For this review, take the finished solid that the model builds, in its own axes (mm). Face numbers are marked on the shaded views. A direction names the side the tool comes from. Give positions to 0.01 mm unless a question says otherwise; leave off trailing zeros. Write each loop counter-clockwise with the first axis right and the second up, starting at its lowest first coordinate (ties: lowest second). Pieces come first, ordered by that corner, then holes.
1) Draft analysis for pull direction Z (two halves, no side actions). For the marked faces 4, 5, 6 and 7, state which applies: pulls with the +Z half, pulls with the -Z half, needs draft (parallel to the pull), parting line crosses it, or undercut.
2) Wall thickness on line 1 along Y through (x, z) = (-24, 11); line 2 along X through (y, z) = (-27, 26.5); line 3 along X through (y, z) = (-14, 32): over which ranges is each line inside the solid? List them lowest first.
3) We need section C-C on x = -18.25. Give the boundary of the cut face in (y, z), and give its area (3 significant figures).
4) We need section B-B on z = 11. Give the boundary of the cut face in (x, y), and give its area (3 significant figures).
5) We need section D-D on y = -26.5. Give the boundary of the cut face in (x, z).
6) For P1, Ø3, axis at x = -16.5, y = -8.5, coming from the +Z side; P2, Ø12, axis at y = -13, z = 28, coming from the -X side; P3, Ø1, axis at y = -11, z = 10, coming from the -X side, all flat-tipped, find the tip position at first contact; note any pin that passes through.
7) Machinability: for the marked faces 1, 2 and 3, which of the approach directions +Z, -Z, +X, -X, +Y, -Y give a long, thin tool a straight path to every point of the face, cutting with its end or side? Answer none if there is none.
8) We need section A-A on y = -37. Give the boundary of the cut face in (x, z).
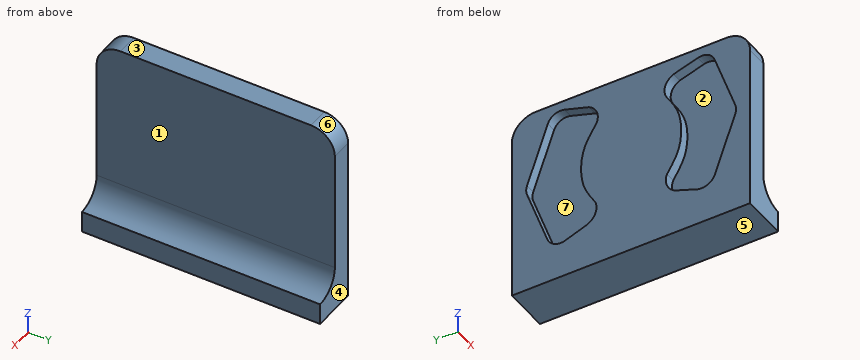
from build123d import *

# Parameters (mm, degrees)
F1_DEPTH = 50
F2_R     = 5
F3_R     = 5
F5_DEPTH = 2.1


with BuildPart() as f1:
    # F0 (on Front) → F1 (new body)
    with BuildSketch(Plane.XZ):
        with BuildLine():
            Line((-24.7697359324, 0), (-15.2697359324, 0))
            Line((-15.2697359324, 0), (-15.2697359324, 4.5))
            ThreePointArc((-15.2697359324, 4.5), (-18.8052698383, 5.9644660941), (-20.2697359324, 9.5))
            Line((-20.2697359324, 9.5), (-20.2697359324, 40))
            Line((-20.2697359324, 40), (-24.7697359324, 40))
            Line((-24.7697359324, 40), (-24.7697359324, 0))
        make_face()
    extrude(amount=F1_DEPTH)

    # F2
    f2_edges = [f1.edges().sort_by_distance(p)[0] for p in [
        (-22.519736, -50, 40),
    ]]
    fillet(f2_edges, radius=F2_R)

    # F3
    f3_edges = [f1.edges().sort_by_distance(p)[0] for p in [
        (-22.519736, 0, 40),
    ]]
    fillet(f3_edges, radius=F3_R)

    # F4 (on face) → F5 (cut)
    with BuildSketch(Plane(origin=(-24.7697359324, 0, 0), x_dir=(0, -1, 0), z_dir=(-1, 0, 0))):
        with BuildLine():
            Line((46.8955885446, 23.8107649305), (42.5171071131, 36.1752150642))
            ThreePointArc((42.5171071131, 36.1752150642), (41.1165449237, 37.7616933331), (39.0073708388, 37.93452974))
            Line((39.0073708388, 37.93452974), (33.9392572641, 36.3604687154))
            ThreePointArc((33.9392572641, 36.3604687154), (32.1739564338, 34.3397574907), (32.4926399743, 31.675549977))
            add(Edge.make_bspline(
                [(32.4926399743, 31.675549977), (33.3670492771, 30.3381403961), (35.0987739091, 27.6894664778), (35.7199990478, 23.1066149427), (35.2211127015, 18.2107984297), (33.4472667585, 15.4309330693), (32.5552672148, 14.0330446884)],
                knots=[0, 0, 0, 0, 0.2493081883, 0.4937426091, 0.7454224458, 1, 1, 1, 1], degree=3))
            ThreePointArc((32.5552672148, 14.0330446884), (32.5347631708, 11.4606329376), (34.2782102525, 9.5690423623))
            Line((34.2782102525, 9.5690423623), (39.1331128776, 7.7970703132))
            ThreePointArc((39.1331128776, 7.7970703132), (41.2400733133, 8.0993579825), (42.6161779425, 9.723241033))
            Line((42.6161779425, 9.723241033), (46.8955885446, 21.8079237751))
            ThreePointArc((46.8955885446, 21.8079237751), (47.0676640713, 22.8093443528), (46.8955885446, 23.8107649305))
        make_face()
        with BuildLine():
            ThreePointArc((3.1705893979, 23.8107653384), (2.9985138712, 22.8093447607), (3.1705893979, 21.807924183))
            Line((3.1705893979, 21.807924183), (7.45, 9.723241441))
            ThreePointArc((7.45, 9.723241441), (8.8261046292, 8.0993583904), (10.9330650649, 7.7970707212))
            Line((10.9330650649, 7.7970707212), (15.78796769, 9.5690427702))
            ThreePointArc((15.78796769, 9.5690427702), (17.5314147718, 11.4606333455), (17.5109107277, 14.0330450963))
            add(Edge.make_bspline(
                [(17.5735379682, 31.6755503849), (16.6991286655, 30.3381408041), (14.9674040335, 27.6894668857), (14.3461788947, 23.1066153507), (14.8450652411, 18.2107988376), (16.618911184, 15.4309334772), (17.5109107277, 14.0330450963)],
                knots=[0, 0, 0, 0, 0.2493081883, 0.4937426091, 0.7454224458, 1, 1, 1, 1], degree=3))
            ThreePointArc((17.5735379682, 31.6755503849), (17.8922215087, 34.3397578986), (16.1269206784, 36.3604691233))
            Line((16.1269206784, 36.3604691233), (11.0588071037, 37.9345301479))
            ThreePointArc((11.0588071037, 37.9345301479), (8.9496330188, 37.7616937411), (7.5490708294, 36.1752154721))
            Line((7.5490708294, 36.1752154721), (3.1705893979, 23.8107653384))
        make_face()
    extrude(amount=-F5_DEPTH, mode=Mode.SUBTRACT)


solid = f1.part
Results list:
1. face 4: needs draft
1. face 5: pulls with the -Z half
1. face 6: pulls with the +Z half
1. face 7: undercut
2. line 1: y = -50 to -43.07, -32.75 to -17.31, -7 to 0
2. line 2: x = -24.77 to -20.27
2. line 3: x = -22.67 to -20.27
3. outline: (-50, 0) - (0, 0) - (0, 5.49) - (-50, 5.49) - close
3. area: 274 mm2
4. outline: (-24.77, -50) - (-20.27, -50) - (-20.27, 0) - (-24.77, 0) - (-24.77, -7) - (-22.67, -7) - (-22.67, -17.31) - (-24.77, -17.31) - (-24.77, -32.75) - (-22.67, -32.75) - (-22.67, -43.07) - (-24.77, -43.07) - close
4. area: 182 mm2
5. outline: (-24.77, 0) - (-15.27, 0) - (-15.27, 4.5) arc R5 cw to (-20.27, 9.5) - (-20.27, 40) - (-24.77, 40) - close
6. P1: stops at z = 5.31
6. P2: stops at x = -24.77
6. P3: stops at x = -22.67
7. face 1: +Z, +X, +Y, -Y
7. face 2: -X
7. face 3: +Z, +X, -X, +Y, -Y
8. outline: (-24.77, 0) - (-15.27, 0) - (-15.27, 4.5) arc R5 cw to (-20.27, 9.5) - (-20.27, 40) - (-24.77, 40) - (-24.77, 37.31) - (-22.67, 37.31) - (-22.67, 8.58) - (-24.77, 8.58) - close
